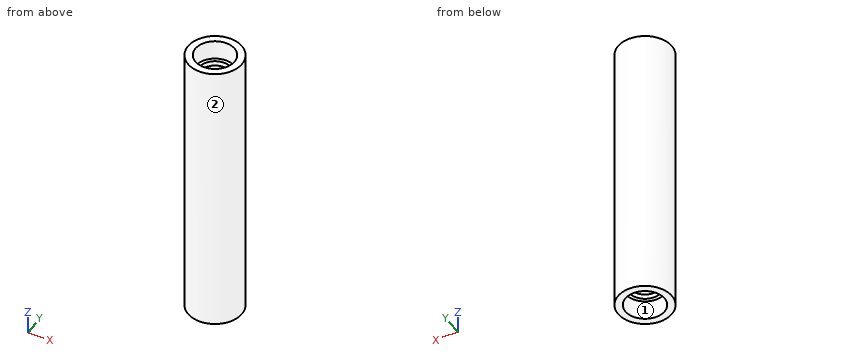
from build123d import *

# Parameters (mm, degrees)
SKETCH1_R           = 11
SKETCH1_R_2         = 8
BOSS_EXTRUDE1_DEPTH = 57.5
BOSS_EXTRUDE2_START = 47.5
SKETCH2_R           = 8
SKETCH2_R_2         = 6.5
BOSS_EXTRUDE2_DEPTH = 2


with BuildPart() as part:
    # Sketch1 → Boss-Extrude1 (new, symmetric)
    with BuildSketch(Plane.XY):
        Circle(SKETCH1_R)
        Circle(SKETCH1_R_2, mode=Mode.SUBTRACT)
    extrude(amount=BOSS_EXTRUDE1_DEPTH, both=True)

    # Sketch2 → Boss-Extrude2 (add)
    with BuildSketch(Plane.XY.offset(BOSS_EXTRUDE2_START)):
        Circle(SKETCH2_R)
        Circle(SKETCH2_R_2, mode=Mode.SUBTRACT)
    boss_extrude2 = extrude(amount=BOSS_EXTRUDE2_DEPTH)

    # Mirror1: Boss-Extrude2 across plane
    add(boss_extrude2.mirror(Plane.XY))


solid = part.part
Verification items for the finished model (mm, model axes). Face numbers are marked on the shaded views. Give positions to 0.01 mm unless a question says otherwise; leave off trailing zeros. Loops run counter-clockwise (first coordinate to the right, second up) from the corner with the lowest first, then second, coordinate; pieces in that order, holes last. Notation, with made-up numbers: (83, 77.25) - (120, 77.25) arc R21 cw to (120, 84.25) - close; hole circle Ø9 at (-6.75, -19). An arc over 180 degrees is marked (long way). Write item = value, one per line. Start each with the question number.
Q1. Depth check by flat-ended pin: P1, Ø8, axis at x = -5, y = 5.5, coming from the +Z side; P2, Ø4, axis at y = -3, z = 1, coming from the +X side; P3, Ø8, axis at x = -7, z = -26, coming from the -Y side; P4, Ø1.5, axis at y = 7, z = -16.5, coming from the -X side. Enter the tip coordinate at first touch or a pass-through.
Q2. Cross-section at A-A, the plane y = 0. Enter the section's corners in (x, z), and give its area (3 significant figures).
Q3. Cross-section at C-C, the plane z = 22. Enter the section's corners in (x, y), and give its area (3 significant figures).
Q4. Mould release check, pull along Y, two halves, no side actions. Record for the marked faces 1 and 2: released by +Y, released by -Y, zero draft, split by the parting line, or undercut.
Q5. Thickness scan on line 1 (Z direction, x = -0.5, y = -7.25); line 2 (Y direction, x = 0, z = -25.5); line 3 (Y direction, x = 0, z = -47.95). Record the ranges inside material, lowest first.
Answer key:
q1.P1 = 57.5
q1.P2 = 10.95
q1.P3 = -10.58
q1.P4 = -9.05
q2.outline = (-11, -57.5) - (-8, -57.5) - (-8, -49.5) - (-6.5, -49.5) - (-6.5, -47.5) - (-8, -47.5) - (-8, 47.5) - (-6.5, 47.5) - (-6.5, 49.5) - (-8, 49.5) - (-8, 57.5) - (-11, 57.5) - close; (6.5, -49.5) - (8, -49.5) - (8, -57.5) - (11, -57.5) - (11, 57.5) - (8, 57.5) - (8, 49.5) - (6.5, 49.5) - (6.5, 47.5) - (8, 47.5) - (8, -47.5) - (6.5, -47.5) - close
q2.area = 702 mm^2
q3.outline = circle Ø22 at (0, 0); hole circle Ø16 at (0, 0)
q3.area = 179 mm^2
q4.face_1 = undercut
q4.face_2 = split by the parting line
q5.line_1 = -49.5 to -47.5, 47.5 to 49.5
q5.line_2 = -11 to -8, 8 to 11
q5.line_3 = -11 to -6.5, 6.5 to 11
